Geometry: final body of the model. Coordinates: model frame, mm. A direction names the side the tool comes from. Give positions to 0.01 mm unless a question says otherwise; leave off trailing zeros. Write each loop counter-clockwise with the first axis right and the second up, starting at its lowest first coordinate (ties: lowest second). Pieces come first, ordered by that corner, then holes. Notation, with made-up numbers: (60.5, 22.5) - (114.5, 22.5) arc R13 cw to (114.5, 35.5) - close; hole circle Ø11 at (73, 63). An arc over 180 degrees is marked (long way). Use CSV: the item, a comma, the result in double quotes. Start each with the question number.
(1) Section A-A on z = -0.5. Output: boundary loops of the cut face in (x, y).
(2) Section B-B on y = 2.5. Output: boundary loops of the cut face in (x, z), and give its area (3 significant figures).
(3) Reachability of faces 1 (the cylindrical face through (3.16, 2.05, -4.48)), 2 (the flat face through (3, 6, 10)), 3 (the flat face through (3, 16, 14.203)), 4 (the flat face through (3.155, 12.727, 3.96)), 5 (the flat face through (3.2, 10.971, -9.4)) from +Z, -Z, +X, -X, +Y, -Y: full face, straight path, thin tool, end or side. Return the list, or none.
(4) First-contact query: pin 1 Ø1.5 at (x, z) = (5.5, 6.5) entering from +Y; pin 2 Ø2 at (x, z) = (1, 3) entering from +Y; pin 3 Ø2.5 at (x, y) = (3, 16) entering from -Z. Flat tips, straight axial feed; report the tip coordinate or a pass-through.
(5) Line query: probe 1 along Y at (x, z) = (4, -4.75); probe 2 along Z at (x, y) = (1.75, 3.5); probe 3 along Z at (x, y) = (2, 2.5). Output: solid intervals per line, ascending. Write a range as [from, to].
(6) Section D-D on z = -4.75. Output: boundary loops of the cut face in (x, y).
(7) Section C-C on x = 1.25. Output: boundary loops of the cut face in (y, z).
from build123d import *

# Parameters (mm, degrees)
SKETCH_1_R      = 1.25
EXTRUDE_1_DEPTH = 6.4


with BuildPart() as part:
    # 草图1 → 凸台-拉伸1 (new body)
    with BuildSketch(Plane(origin=(0, 0, 0), x_dir=(0, 0, -1), z_dir=(1, 0, 0))):
        with BuildLine():
            Line((-10, 10.970845222), (6, 10.970845222))
            Line((6, 10.970845222), (-14.202813689, 14.533146362))
            Line((-14.202813689, 14.533146362), (-14.202813689, 17.533146362))
            ThreePointArc((-14.202813689, 17.533146362), (-12.796398802, 18.939561248), (-11.389983916, 17.533146362))
            Line((-11.389983916, 17.533146362), (-11.389983916, 14.544881886))
            Line((-11.389983916, 14.544881886), (8.879385242, 10.970845222))
            Line((8.879385242, 10.970845222), (10, 10.970845222))
            Line((10, 10.970845222), (10, 0.770845222))
            Line((10, 0.770845222), (-10, 0.770845222))
            Line((-10, 0.770845222), (-10, 10.970845222))
        make_face()
        with Locations((-4.75, 3.270845222)):
            Circle(SKETCH_1_R, mode=Mode.SUBTRACT)
        with Locations((4.75, 3.270845222)):
            Circle(SKETCH_1_R, mode=Mode.SUBTRACT)
    extrude(amount=EXTRUDE_1_DEPTH)


solid = part.part
Check values:
1,outline,"(0, 0.77) - (6.4, 0.77) - (6.4, 10.97) - (0, 10.97) - close; (0, 11.94) - (6.4, 11.94) - (6.4, 12.45) - (0, 12.45) - close"
2,outline,"(0, -10) - (6.4, -10) - (6.4, -5.73) - (0, -5.73) - close; (0, -3.77) - (6.4, -3.77) - (6.4, 3.77) - (0, 3.77) - close; (0, 5.73) - (6.4, 5.73) - (6.4, 10) - (0, 10) - close"
2,area,"103 mm²"
3,face 1,"+X, -X"
3,face 2,"+Z, +X, -X, -Y"
3,face 3,"+Z, +X, -X, +Y, -Y"
3,face 4,"+Z, +X, -X"
3,face 5,"-Z, +X, -X, +Y"
4,pin 1,"stops at y = 13.81"
4,pin 2,"stops at y = 13.24"
4,pin 3,"stops at z = 11.39"
5,probe 1,"y = [0.77, 2.02], [4.52, 10.97], [11.19, 11.7]"
5,probe 2,"z = [-10, -5.98], [-3.52, 3.52], [5.98, 10]"
5,probe 3,"z = [-10, -5.73], [-3.77, 3.77], [5.73, 10]"
6,outline,"(0, 0.77) - (6.4, 0.77) - (6.4, 2.02) - (0, 2.02) - close; (0, 4.52) - (6.4, 4.52) - (6.4, 10.97) - (0, 10.97) - close; (0, 11.19) - (6.4, 11.19) - (6.4, 11.7) - (0, 11.7) - close"
7,outline,"(0.77, -10) - (10.97, -10) - (10.97, -8.88) - (14.54, 11.39) - (17.53, 11.39) arc R1.41 ccw to (17.53, 14.2) - (14.53, 14.2) - (10.97, -6) - (10.97, 10) - (0.77, 10) - close; hole circle Ø2.5 at (3.27, -4.75); hole circle Ø2.5 at (3.27, 4.75)"
